Design review of the part built by this model. Coordinates are the model's own, in mm. Face numbers are marked on the shaded views. A direction names the side the tool comes from. Give positions to 0.01 mm unless a question says otherwise; leave off trailing zeros. Loops run counter-clockwise (first coordinate to the right, second up) from the corner with the lowest first, then second, coordinate; pieces in that order, holes last. Notation, with made-up numbers: (76.25, 11.5) -> (116.25, 11.5) arc R10 ccw to (116.25, 30.5) -> close; hole circle Ø7 at (-4, -28). An arc over 180 degrees is marked (long way). Answer in a Markdown table with one row per item. Add a question column.
(1) Consider section D-D on z = 0. Write out the cut boundary in (x, y).
(2) For line 1 (X direction, y = -87.5, z = 66.5); line 2 (Y direction, x = -29, z = 0); line 3 (Z direction, x = -5, y = -84.5), list the stretches that pass through material, from the lowest coordinate up.
(3) Consider section A-A on y = 33.5. Write out the cut boundary in (x, z), then the cut area to 3 significant figures.
(4) Consider section B-B on z = 84. Write out the cut boundary in (x, y).
(5) For pin 1 (5 mm diameter, centred on x = -8.5, y = -101.5, fed in from -Z); pin 2 (12 mm diameter, centred on x = -5.5, z = -4, fed in from +Y); pin 3 (12 mm diameter, centred on x = -8.5, y = 45, fed in from +Z); pin 4 (12 mm diameter, centred on y = 0, z = 0, fed in from +X), all flat-tipped, find the tip position at first contact; note any pin that passes through.
(6) Consider section C-C on x = -35. Write out the cut boundary in (y, z), then the cut area to 3 significant figures.
(7) For the marked faces 1, 2 and 3, list the 3-axis set-ups (+Z, -Z, +X, -X, +Y, -Y) from which the entire face can be reached by the end or side of a thin tool; tool diameter is ignored.
from build123d import *

# Parameters (mm, degrees)
SKETCH_4_W          = 38
SKETCH_4_H          = 58
EXTRUDE_1_DEPTH     = 15
EXTRUDE_START       = -2
EXTRUDE_2_DEPTH     = 10
EXTRUDE_3_DEPTH     = 15
SKETCH_8_R          = 19.2
EXTRUDE_4_DEPTH     = 15
RIB_4_REACH         = 173.764
SKETCH_7_WALL_W     = 417.368166338
SKETCH_7_WALL_H     = 10
RIB_4_DRAFT_ANGLE   = 0.1993373
SKETCH_9_R          = 10
CUT_EXTRUDE_1_DEPTH = 172.764033058
SKETCH_10_W         = 25
SKETCH_10_H         = 28
CUT_EXTRUDE_2_DEPTH = 169.724281158


with BuildPart() as part:
    # Sketch 4 → Extrude 1 (new body)
    with BuildSketch(Plane(origin=(0, 0, 0), x_dir=(0, 0, -1), z_dir=(1, 0, 0))):
        with Locations((0, 29)):
            Rectangle(SKETCH_4_W, SKETCH_4_H)
    extrude(amount=-EXTRUDE_1_DEPTH)

    # Sketch 2 → Revolve 1 (revolve)
    with BuildSketch(Plane.XY, mode=Mode.PRIVATE) as revolve_1_sk:
        Polygon((-42, 0), (-42, 15), (0, 19.2), (0, 0), align=None)
    revolve(revolve_1_sk.sketch.rotate(Axis((-18.865866606, 0, 0), (1, 0, 0)), 90), axis=Axis((-18.865866606, 0, 0), (1, 0, 0)))



with BuildPart() as body_2:
    # Sketch 5 → Extrude 2 (new body)
    with BuildSketch(Plane(origin=(0, 0, 0), x_dir=(0, 0, -1), z_dir=(1, 0, 0)).offset(EXTRUDE_START)):
        with BuildLine():
            Line((-111.66423124, -79.82543117), (-102.463778118, -87.579530564))
            ThreePointArc((-102.463778118, -87.579530564), (-72.822222222, -86.405578238), (-68.958444104, -115.817671306))
            Line((-68.958444104, -115.817671306), (-59.757990982, -123.5717707))
            Line((-59.757990982, -123.5717707), (-58.756458022, -122.156778939))
            Line((-58.756458022, -122.156778939), (15.949294293, -10.689247473))
            ThreePointArc((15.949294293, -10.689247473), (-5.586302425, -18.369355602), (-19.2, 0))
            ThreePointArc((-19.2, 0), (-20.177119331, -4.311336735), (-22.917524888, -7.780135376))
            Line((-22.917524888, -7.780135376), (-108.360415381, -76.775442927))
            Line((-108.360415381, -76.775442927), (-111.66423124, -79.82543117))
        make_face()
    extrude(amount=-EXTRUDE_2_DEPTH)

    # Sketch 6 → Extrude 3 (add)
    with BuildSketch(Plane(origin=(0, 0, 0), x_dir=(0, 0, -1), z_dir=(1, 0, 0))):
        with BuildLine():
            Line((-111.66423124, -79.82543117), (-102.463778118, -87.579530564))
            ThreePointArc((-102.463778118, -87.579530564), (-72.822222222, -86.405578238), (-68.958444104, -115.817671306))
            Line((-68.958444104, -115.817671306), (-59.757990982, -123.5717707))
            ThreePointArc((-59.757990982, -123.5717707), (-65.088888889, -77.22976462), (-111.66423124, -79.82543117))
        make_face()
    extrude(amount=-EXTRUDE_3_DEPTH)


with BuildPart() as part_1:
    add(part.part)

    add(body_2.part)  # Extrude 4 merges body 2
    # Sketch 8 → Extrude 4 (add)
    with BuildSketch(Plane(origin=(0, 0, 0), x_dir=(0, 0, -1), z_dir=(1, 0, 0))):
        Circle(SKETCH_8_R)
    extrude(amount=-EXTRUDE_4_DEPTH)

    # Sketch 7 wall → Rib 4 (add, up to next)
    with BuildSketch(Plane(origin=(-22, -38.61488231, 32.544444445), x_dir=(0.278396048141, -0.734421696805, 0.618967213705), z_dir=(0.960466366084, 0.212875854148, -0.17941078658)), mode=Mode.PRIVATE) as rib_4_sk1:
        Rectangle(SKETCH_7_WALL_W, SKETCH_7_WALL_H)
    rib_4_tool1 = extrude(rib_4_sk1.sketch, amount=RIB_4_REACH, mode=Mode.PRIVATE) - part_1.part
    add(rib_4_tool1.solids().sort_by_distance((-22, -38.61488231, 32.544444445))[0])

    # Rib 4 draft
    rib_4_draft_faces = [part_1.faces().sort_by_distance(p)[0] for p in [
        (-21.519766817, -41.730666605, 28.631483377),
        (-21.519766817, -35.286222161, 36.277994725),
    ]]
    draft(rib_4_draft_faces, Plane(origin=(-22, -38.61488231, 32.544444445), x_dir=(0.278396048141, -0.734421696805, 0.618967213705), z_dir=(-0.960466366084, -0.212875854148, 0.17941078658)), RIB_4_DRAFT_ANGLE)

    # Sketch 9 → Cut-Extrude 1 (cut, through all)
    with BuildSketch(Plane.ZY.offset(42)):
        Circle(SKETCH_9_R)
    extrude(amount=-CUT_EXTRUDE_1_DEPTH, mode=Mode.SUBTRACT)

    # Sketch 10 → Cut-Extrude 2 (cut, through all)
    with BuildSketch(Plane.ZY.offset(15)):
        with Locations((0, 44)):
            Rectangle(SKETCH_10_W, SKETCH_10_H)
    extrude(amount=-CUT_EXTRUDE_2_DEPTH, mode=Mode.SUBTRACT)


solid = part_1.part
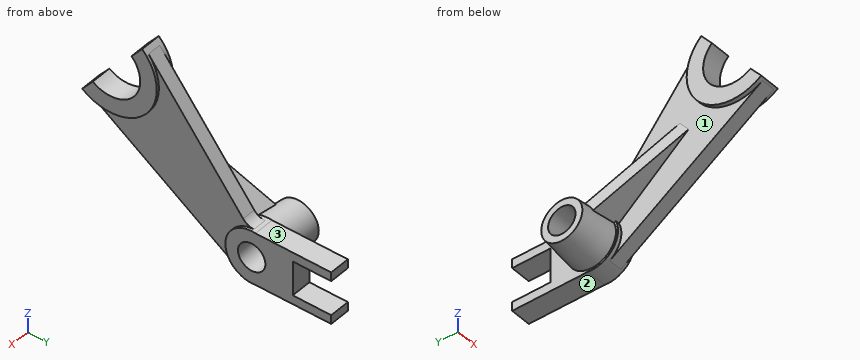
Values follow:
| question | item | result |
|---|---|---|
| 1 | outline | (-42, -15) -> (-15, -17.7) -> (-15, -19.2) -> (-12, -19.2) -> (-12, -34.49) -> (-2, -34.49) -> (-2, -19.2) -> (0, -19.2) -> (0, -10) -> (-42, -10) -> close; (-42, 10) -> (0, 10) -> (0, 30) -> (-15, 30) -> (-15, 17.7) -> (-42, 15) -> close |
| 2 | line 1 | -15 to 0 |
| 2 | line 2 | -16.3 to -10, 10 to 16.3 |
| 2 | line 3 | 33.52 to 75.46, 98.54 to 106.12 |
| 3 | outline | (-15, -19) -> (0, -19) -> (0, -12.5) -> (-15, -12.5) -> close; (-15, 12.5) -> (0, 12.5) -> (0, 19) -> (-15, 19) -> close |
| 3 | area | 195 mm2 |
| 4 | outline | (-15, -81.43) -> (0, -81.43) -> (0, -69.36) -> (-2, -69.36) -> (-2, -57.1) -> (-12, -57.1) -> (-12, -69.36) -> (-15, -69.36) -> close |
| 5 | pin 1 | z = 43.24 |
| 5 | pin 2 | y = 30 |
| 5 | pin 3 | z = 19 |
| 5 | pin 4 | through |
| 6 | outline | circle Ø31.4 at (0, 0); hole circle Ø20 at (0, 0) |
| 6 | area | 460 mm2 |
| 7 | face 1 | -X |
| 7 | face 2 | -Z, +X, -X, +Y |
| 7 | face 3 | +Z, +X, -X, +Y |
